from build123d import *

# Parameters (mm, degrees)
SKETCH1_W           = 50.8
SKETCH1_H           = 25.4
SKETCH1_W_2         = 45.72
SKETCH1_H_2         = 20.32
EXTRUDE_THIN1_DEPTH = 113.411
SKETCH2_R           = 1.3589
CUT_EXTRUDE1_DEPTH  = 51.8
LPATTERN1_COUNT     = 9
LPATTERN1_PITCH     = 25.4


with BuildPart() as part:
    # Sketch1 → Extrude-Thin1 (new body, symmetric)
    with BuildSketch(Plane.XY):
        Rectangle(SKETCH1_W, SKETCH1_H)
        Rectangle(SKETCH1_W_2, SKETCH1_H_2, mode=Mode.SUBTRACT)
    extrude(amount=EXTRUDE_THIN1_DEPTH, both=True)

    # Sketch2 → Cut-Extrude1 (cut, through all)
    with BuildSketch(Plane(origin=(25.4, 0, 0), x_dir=(0, 0, -1), z_dir=(1, 0, 0))):
        with Locations((-100.711, 0)):
            Circle(SKETCH2_R)
    cut_extrude1 = extrude(amount=-CUT_EXTRUDE1_DEPTH, mode=Mode.SUBTRACT)

    # LPattern1: Cut-Extrude1 ×9
    with Locations(*[(0, 0, -i * LPATTERN1_PITCH) for i in range(1, LPATTERN1_COUNT)]):
        add(cut_extrude1, mode=Mode.SUBTRACT)


solid = part.part
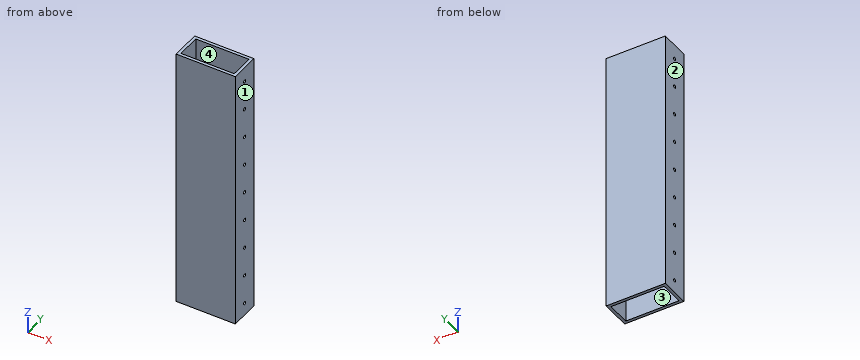
Source: CAD feature listing. Evaluate the final solid. Frame: model axes, mm. Face numbers are marked on the shaded views. Give positions to 0.01 mm unless a question says otherwise; leave off trailing zeros. Loops run counter-clockwise (first coordinate to the right, second up) from the corner with the lowest first, then second, coordinate; pieces in that order, holes last. Notation, with made-up numbers: (-9, -2.75) -> (27, -2.75) arc R18 ccw to (27, 6.25) -> close; hole circle Ø10 at (68.25, 45). An arc over 180 degrees is marked (long way). Use a Markdown table: item, result. Add a question column.
1) Section query C-C, the plane x = 9. Return the cut outline in (y, z).
2) Pull-direction query (X, two-part tool) for the marked faces 1, 2, 3 and 4; classes: +X half, -X half, draft (parallel to the pull), parting line (faces both ways), or undercut.
3) Section query A-A, the plane y = -4.5. Return the cut outline in (x, z).
4) Section query B-B, the plane z = 87. Return the cut outline in (x, y), then the cut area to 3 significant figures.
5) Line query: line 1 along X through (y, z) = (-6.5, -91); line 2 along Y through (x, z) = (-18, 83). Output: solid intervals per line, ascending. Write a range as [from, to].
6) First-contact query: pin 1 (4.5 mm diameter, centred on y = 0, z = 100.711, fed in from +X). Flat tip, straight axial feed; report the tip coordinate or a pass-through.
Numbers:
| question | item | result |
|---|---|---|
| 1 | outline | (-12.7, -113.41) -> (-10.16, -113.41) -> (-10.16, 113.41) -> (-12.7, 113.41) -> close; (10.16, -113.41) -> (12.7, -113.41) -> (12.7, 113.41) -> (10.16, 113.41) -> close |
| 2 | face 1 | +X half |
| 2 | face 2 | -X half |
| 2 | face 3 | undercut |
| 2 | face 4 | undercut |
| 3 | outline | (-25.4, -113.41) -> (-22.86, -113.41) -> (-22.86, 113.41) -> (-25.4, 113.41) -> close; (22.86, -113.41) -> (25.4, -113.41) -> (25.4, 113.41) -> (22.86, 113.41) -> close |
| 4 | outline | (-25.4, -12.7) -> (25.4, -12.7) -> (25.4, 12.7) -> (-25.4, 12.7) -> close; hole (-22.86, -10.16) -> (22.86, -10.16) -> (22.86, 10.16) -> (-22.86, 10.16) -> close |
| 4 | area | 361 mm2 |
| 5 | line 1 | x = [-25.4, -22.86], [22.86, 25.4] |
| 5 | line 2 | y = [-12.7, -10.16], [10.16, 12.7] |
| 6 | pin 1 | stops at x = 25.4 |
